```python
from build123d import *

# Parameters (mm, degrees)
F0_R     = 71
F1_DEPTH = 1.7
F2_R     = 69
F3_DEPTH = 1.6
F4_R     = 31.25
F5_DEPTH = 25


with BuildPart() as f1:
    # F0 (on Top) → F1 (new body)
    with BuildSketch(Plane.XY):
        Circle(F0_R)
    extrude(amount=F1_DEPTH)

    # F2 (on face) → F3 (join)
    with BuildSketch(Plane.XY.offset(1.7)):
        Circle(F2_R)
    extrude(amount=F3_DEPTH)

    # F4 (on face) → F5 (cut)
    with BuildSketch(Plane.XY.offset(3.3)):
        with Locations((29.75, 0)):
            Circle(F4_R)
    extrude(amount=-F5_DEPTH, mode=Mode.SUBTRACT)


solid = f1.part
```
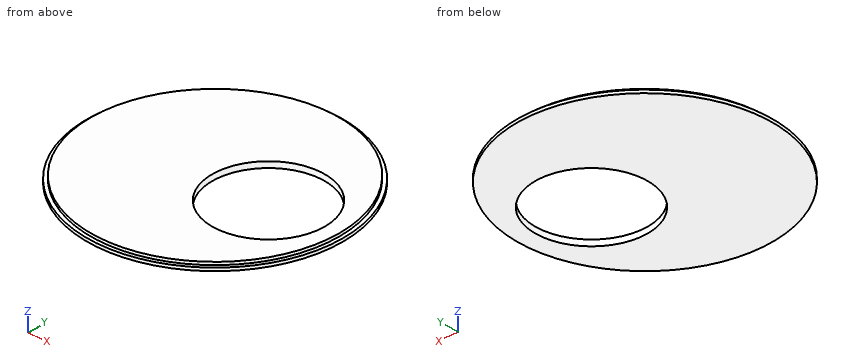
Geometry check sheet. Reference: the model listing, model coordinates, mm. Give positions to 0.01 mm unless a question says otherwise; leave off trailing zeros. Write each loop counter-clockwise with the first axis right and the second up, starting at its lowest first coordinate (ties: lowest second). Pieces come first, ordered by that corner, then holes. Notation, with made-up numbers: (57.5, 45) -> (116.5, 45) arc R18 ccw to (116.5, 77) -> close; hole circle Ø4 at (41, 34). An arc over 180 degrees is marked (long way). Use one line per item in the form item = value.
Item 1: Sectioned sample at C-C on z = 2.4. Enter the section's corners in (x, y).
Results list:
outline = circle Ø138 at (0, 0); hole circle Ø62.5 at (29.75, 0)
Item 2: Sectioned sample at D-D on x = -12. Enter the section's corners in (y, z).
Results list:
outline = (-69.98, 0) -> (69.98, 0) -> (69.98, 1.7) -> (67.95, 1.7) -> (67.95, 3.3) -> (-67.95, 3.3) -> (-67.95, 1.7) -> (-69.98, 1.7) -> close
Item 3: Depth check by flat-ended pin: pin 1 Ø1.5 at (x, z) = (19, 1.5) entering from -Y. Enter the tip coordinate at first touch or a pass-through.
Results list:
pin_1 = -68.61
Item 4: Sectioned sample at B-B on x = 29.75. Enter the section's corners in (y, z).
Results list:
outline = (-64.47, 0) -> (-31.25, 0) -> (-31.25, 3.3) -> (-62.26, 3.3) -> (-62.26, 1.7) -> (-64.47, 1.7) -> close; (31.25, 0) -> (64.47, 0) -> (64.47, 1.7) -> (62.26, 1.7) -> (62.26, 3.3) -> (31.25, 3.3) -> close
Item 5: Scan lines: line 1 (Y direction, x = 29.75, z = 0.85); line 2 (Y direction, x = 12.5, z = 2.45); line 3 (X direction, y = -29, z = 0.9). Record each from-to range of solid material in increasing order.
Results list:
line_1 = -64.47 to -31.25, 31.25 to 64.47
line_2 = -67.86 to -26.06, 26.06 to 67.86
line_3 = -64.81 to 18.11, 41.39 to 64.81
Item 6: Sectioned sample at A-A on y = 0. Enter the section's corners in (x, z), plus the area to 3 significant figures.
Results list:
outline = (-71, 0) -> (-1.5, 0) -> (-1.5, 3.3) -> (-69, 3.3) -> (-69, 1.7) -> (-71, 1.7) -> close; (61, 0) -> (71, 0) -> (71, 1.7) -> (69, 1.7) -> (69, 3.3) -> (61, 3.3) -> close
area = 256 mm2
